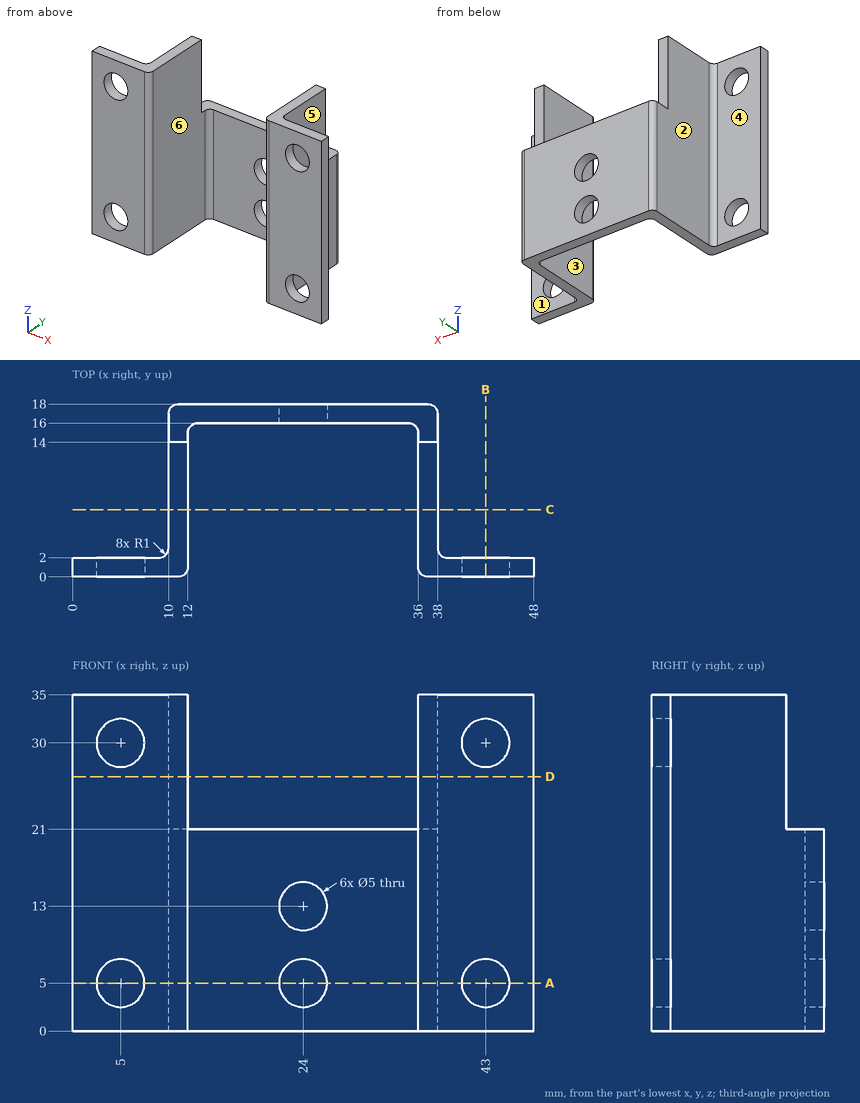
Geometry check sheet. Reference: drawing and pictorial views, mm from the part's lowest x, y, z. A direction names the side the tool comes from. Round coordinates to 2 decimals unless told otherwise and drop trailing zeros. Loops run counter-clockwise (first coordinate to the right, second up) from the corner with the lowest first, then second, coordinate; pieces in that order, holes last. Notation, with made-up numbers: (25, -34) -> (83, -34) arc R16 cw to (83, -25) -> close; hole circle Ø3 at (72.25, 46). An arc over 180 degrees is marked (long way). Answer as a JSON object with one key per item and string values.
Q1. Section check A-A (z = 5). State how many separate pieces and enclosed holes the cut face has, then the cut area to 3 significant figures.
Data:
{"separate pieces": "4", "enclosed holes": "0", "area": "130 mm2"}
Q2. Scan lines: line 1 (Z direction, x = 24, y = 16.7); line 2 (Z direction, x = 5, y = 1.05); line 3 (X direction, y = 9.25, z = 12.5). Record each from-to range of solid material in increasing order. Write a range as from..to.
Data:
{"line 1": "z = 0..2.5, 7.5..10.5, 15.5..21", "line 2": "z = 0..2.5, 7.5..27.5, 32.5..35", "line 3": "x = 10..12, 36..38"}
Q3. Section check C-C (y = 7). Record the boundary of the cut face in (x, z), then the cut area to 3 significant figures.
Data:
{"outline": "(10, 0) -> (12, 0) -> (12, 35) -> (10, 35) -> close; (36, 0) -> (38, 0) -> (38, 35) -> (36, 35) -> close", "area": "140 mm2"}
Q4. Section check D-D (z = 26.5). Record the boundary of the cut face in (x, y), then the cut area to 3 significant figures.
Data:
{"outline": "(0, 0) -> (11, 0) arc R1 ccw to (12, 1) -> (12, 14) -> (10, 14) -> (10, 3) arc R1 cw to (9, 2) -> (0, 2) -> close; (36, 1) arc R1 ccw to (37, 0) -> (48, 0) -> (48, 2) -> (39, 2) arc R1 cw to (38, 3) -> (38, 14) -> (36, 14) -> close", "area": "96.0 mm2"}
Q5. Go/stop test with flat-tipped pins: P1, Ø2, axis at x = 27.5, y = 16, coming from the +Z side; P2, Ø2, axis at x = 33.5, z = 18, coming from the -Y side; P3, Ø6, axis at x = 6.5, y = 8, coming from the +Z side; P4, Ø6, axis at x = 5, z = 30, coming from the +Y side. Record where each tip stops, or that it passes through.
Data:
{"P1": "stops at z = 21", "P2": "stops at y = 16", "P3": "passes through", "P4": "stops at y = 2"}
Q6. Draft check along X on the marked faces 1, 2 and 3. Enter one of: pulls with the +X half, pulls with the -X half, needs draft (parallel to the pull), parting line crosses it, or undercut.
Data:
{"face 1": "needs draft", "face 2": "pulls with the -X half", "face 3": "undercut"}
Q7. Access from +Z, -Z, +X, -X, +Y, -Y to the whole of each face (thin tool, end or side, straight path). Record for the marked faces 4, 5 and 6.
Data:
{"face 4": "+Z, -Z, -X, +Y", "face 5": "+Z, -Z, +X, +Y", "face 6": "+Z, -Z, -Y"}
Q8. Section check B-B (x = 43). Record the boundary of the cut face in (y, z), then the cut area to 3 significant figures.
Data:
{"outline": "(0, 0) -> (2, 0) -> (2, 2.5) -> (0, 2.5) -> close; (0, 7.5) -> (2, 7.5) -> (2, 27.5) -> (0, 27.5) -> close; (0, 32.5) -> (2, 32.5) -> (2, 35) -> (0, 35) -> close", "area": "50.0 mm2"}
